Could you check a few things on this model? Use its own coordinates, in mm. A direction names the side the tool comes from. Coordinates: 2 decimals unless noted, no trailing zeros. Loops run counter-clockwise (first coordinate to the right, second up) from the corner with the lowest first, then second, coordinate; pieces in that order, holes last. Notation, with made-up numbers: (82.25, 47.25) -> (105.25, 47.25) arc R21 ccw to (105.25, 51.25) -> close; hole circle Ø4 at (2, -29.5). An arc over 180 degrees is marked (long way). One line per question, with ' | ' between items.
from build123d import *

# Parameters (mm, degrees)
SKIZZE1_R                       = 10
AUFSATZ_LINEAR_AUSTRAGEN1_DEPTH = 538
SKIZZE2_R                       = 6
AUFSATZ_LINEAR_AUSTRAGEN2_DEPTH = 105
FASE1_SIZE                      = 0.5
CUT_EXTRUDE1_DEPTH              = 2.5


with BuildPart() as part:
    # Skizze1 → Aufsatz-Linear austragen1 (new body)
    with BuildSketch(Plane(origin=(0, 0, 0), x_dir=(1, 0, 0), z_dir=(0, 1, 0))):
        with Locations(Location((0, 0, 0), (0, 0, 270))):  # turned: the seam where the file's is
            Circle(SKIZZE1_R)
    extrude(amount=AUFSATZ_LINEAR_AUSTRAGEN1_DEPTH)

    # Skizze2 → Aufsatz-Linear austragen2 (add)
    with BuildSketch(Plane.XZ):
        with Locations(Location((0, 0, 0), (0, 0, 90))):  # turned: the seam where the file's is
            Circle(SKIZZE2_R)
    extrude(amount=AUFSATZ_LINEAR_AUSTRAGEN2_DEPTH)

    # Fase1
    fase1_edges = [part.edges().sort_by_distance(p)[0] for p in [
        (0, 0, -10),
        (0, 538, -10),
        (0, -105, -6),
    ]]
    chamfer(fase1_edges, length=FASE1_SIZE)

    # Sketch3 → Cut-Extrude1 (cut)
    with BuildSketch(Plane(origin=(1.706808785, -105, 6), x_dir=(0, -1, 0), z_dir=(0, 0, -1))):
        with BuildLine():
            Line((-64, 3.706808785), (-90, 3.706808785))
            ThreePointArc((-90, 3.706808785), (-92, 1.706808785), (-90, -0.293191215))
            Line((-90, -0.293191215), (-64, -0.293191215))
            ThreePointArc((-64, -0.293191215), (-62, 1.706808785), (-64, 3.706808785))
        make_face()
    extrude(amount=CUT_EXTRUDE1_DEPTH, mode=Mode.SUBTRACT)


solid = part.part
1) I need wall thicknesses on line 1 along Z through (x, y) = (-3, 512.5); line 2 along Y through (x, z) = (7.75, 2); line 3 along Z through (x, y) = (0.75, 489). Which ranges of each line are inside material? Lowest first, please. Write a range as from..to.
Data:
line 1: -9.54..9.54 | line 2: 0..538 | line 3: -9.97..9.97
2) If we section it at B-B on y = 59: Please give me the cut outline in (x, z).
Data:
outline: circle Ø20 at (0, 0)
3) On a 3-axis mill with a long thin cutter (end or side, diameter ignored), from which of +Z, -Z, +X, -X, +Y, -Y can I reach the whole of each face in a straight line? I mean faces 1 (the face through (-9.76, 265.24, -2.17)), 2 (the face through (3.65, -51.52, -4.76)). Say none if no direction works.
Data:
face 1: +Y, -Y | face 2: -Y
4) I'm going to push flat-ended pins straight in: pin 1 Ø5 at (x, y) = (5.5, 471) entering from -Z; pin 2 Ø12 at (x, y) = (4, 190.5) entering from +Z; pin 3 Ø1.2 at (x, y) = (0.5, -26) entering from +Z; pin 4 Ø1.7 at (y, z) = (-23.5, 4.5) entering from -X. Where does each tip first touch, or does it pass through?
Data:
pin 1: z = -9.54 | pin 2: z = 10 | pin 3: z = 3.5 | pin 4: x = -4.76
5) If we section it at A-A on z = 0: Please give me the cut outline in (x, y).
Data:
outline: (-10, 0.5) -> (-9.5, 0) -> (-6, 0) -> (-6, -104.5) -> (-5.5, -105) -> (5.5, -105) -> (6, -104.5) -> (6, 0) -> (9.5, 0) -> (10, 0.5) -> (10, 537.5) -> (9.5, 538) -> (-9.5, 538) -> (-10, 537.5) -> close
